```python
from build123d import *

# Parameters (mm, degrees)
BOSS_EXTRUDE1_DEPTH     = 10
BOSS_EXTRUDE2_DEPTH     = 30
BOSS_EXTRUDE3_REACH     = 323.598
CUT_EXTRUDE1_DEPTH      = 396.885084336
CUT_EXTRUDE1_DEPTH_BACK = 396.885084336
SKETCH5_W               = 30
SKETCH5_H               = 30


with BuildPart() as part:
    # Sketch1 → Boss-Extrude1 (new body)
    with BuildSketch(Plane(origin=(0, 0, 0), x_dir=(1, 0, 0), z_dir=(0, 1, 0))):
        with BuildLine():
            Line((-185, -65), (5, -65))
            ThreePointArc((5, -65), (60.514401442, -84.704810384), (91.182336182, -135))
            Line((91.182336182, -135), (185, -135))
            Line((185, -135), (185, 135))
            Line((185, 135), (-185, 135))
            Line((-185, 135), (-185, -65))
        make_face()
    extrude(amount=BOSS_EXTRUDE1_DEPTH)

    # Sketch2 → Boss-Extrude2 (add)
    with BuildSketch(Plane(origin=(0, 10, 0), x_dir=(1, 0, 0), z_dir=(0, 1, 0))):
        Polygon((-175, -35), (-175, 30), (-185, 30), (-185, -45), (-142.5, -45), (-142.5, -35), align=None)
        Polygon((-175, 125), (-142.5, 125), (-142.5, 135), (-185, 135), (-185, 60), (-175, 60), align=None)
        Polygon((-95, -35), (-95, 30), (-85, 30), (-85, -45), (-127.5, -45), (-127.5, -35), align=None)
        Polygon((-127.5, 135), (-127.5, 125), (-95, 125), (-95, 60), (-85, 60), (-85, 135), align=None)
    extrude(amount=BOSS_EXTRUDE2_DEPTH)

    # Boss-Extrude3: up to this face of the body (flat: up to its plane)
    boss_extrude3_end = Plane(part.part.faces().sort_by_distance((-158.75, 25, 35))[0])
    # Sketch3 → Boss-Extrude3 (add, up to the picked face)
    with BuildSketch(Plane.XY.offset(-125), mode=Mode.PRIVATE) as boss_extrude3_sk1:
        with BuildLine():
            ThreePointArc((-134.999999946, 10), (-159.999999978, 18.333333317), (-175, 40))
            Line((-175, 40), (-175, 10))
            Line((-175, 10), (-134.999999946, 10))
        make_face()
    boss_extrude3_tool1 = split(extrude(boss_extrude3_sk1.sketch, amount=BOSS_EXTRUDE3_REACH, mode=Mode.PRIVATE), bisect_by=boss_extrude3_end, keep=Keep.BOTH, mode=Mode.PRIVATE)
    # Sketch3 → Boss-Extrude3 (add, up to the picked face)
    with BuildSketch(Plane.XY.offset(-125), mode=Mode.PRIVATE) as boss_extrude3_sk2:
        with BuildLine():
            Line((-134.999999946, 10), (-95, 10))
            Line((-95, 10), (-95, 40))
            ThreePointArc((-95, 40), (-109.999999978, 18.33333335), (-134.999999946, 10))
        make_face()
    boss_extrude3_tool2 = split(extrude(boss_extrude3_sk2.sketch, amount=BOSS_EXTRUDE3_REACH, mode=Mode.PRIVATE), bisect_by=boss_extrude3_end, keep=Keep.BOTH, mode=Mode.PRIVATE)
    add(boss_extrude3_tool1.solids().sort_by(Axis((-165.840385, 17.926758, -125), (0, 0, 1)))[0])
    add(boss_extrude3_tool2.solids().sort_by(Axis((-104.159615, 17.926758, -125), (0, 0, 1)))[0])

    # Sketch5 → Cut-Extrude1 (cut, two sides: drawn at the far end of the back side and taken through both)
    with BuildSketch(Plane.ZY.offset(185).offset(-CUT_EXTRUDE1_DEPTH_BACK)):
        with Locations((-45, 25)):
            Rectangle(SKETCH5_W, SKETCH5_H)
    extrude(amount=CUT_EXTRUDE1_DEPTH + CUT_EXTRUDE1_DEPTH_BACK, mode=Mode.SUBTRACT)


solid = part.part
```
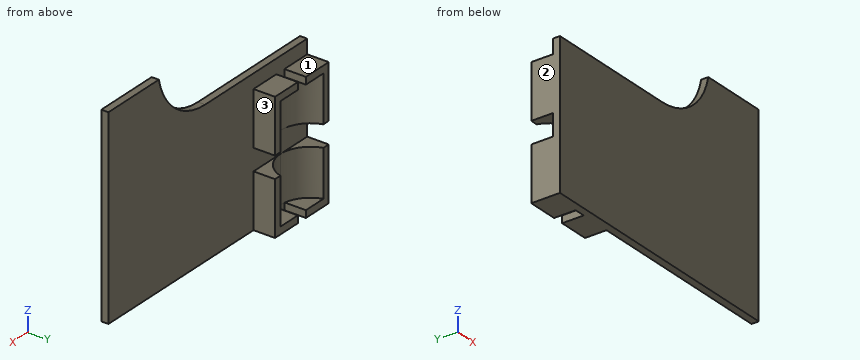
Geometry: final body of the model. Coordinates: model frame, mm. Face numbers are marked on the shaded views. A direction names the side the tool comes from. Coordinates: 2 decimals unless noted, no trailing zeros. Order: outer loops, then holes, each group sorted by start corner. A loop starts at its lowest first (then second) coordinate and runs counter-clockwise, first axis right, second up.
Item 1: Section query D-D (x = 79). Output: boundary loops of the cut face in (y, z), then the cut area to 3 significant figures.
Answer:
outline: (0, -135) - (10, -135) - (10, 105.33) - (0, 105.33) - close
area: 2,400 mm2
Item 2: Section query C-C (x = 118.5). Output: boundary loops of the cut face in (y, z).
Answer:
outline: (0, -135) - (10, -135) - (10, 135) - (0, 135) - close
Item 3: Access query for the marked faces 1, 2 and 3. Directions: +Z, -Z, +X, -X, +Y, -Y. A direction counts if a zero-diameter tool reaches every point of the face in a straight line with its end or side. Return the directions, or none.
Answer:
face 1: +Z, +X, -X, +Y
face 2: +Z, -Z, -X, +Y, -Y
face 3: +Z, -Z, +X, +Y
Item 4: Section query A-A (y = 26.5). Output: boundary loops of the cut face in (x, z), then the cut area to 3 significant figures.
Answer:
outline: (-185, -135) - (-142.5, -135) - (-142.5, -125) - (-168.21, -125) - (-168.21, -60) - (-185, -60) - close; (-185, -30) - (-168.21, -30) - (-168.21, 35) - (-142.5, 35) - (-142.5, 45) - (-185, 45) - close; (-127.5, -135) - (-85, -135) - (-85, -60) - (-101.79, -60) - (-101.79, -125) - (-127.5, -125) - close; (-127.5, 35) - (-101.79, 35) - (-101.79, -30) - (-85, -30) - (-85, 45) - (-127.5, 45) - close
area: 6,070 mm2
Item 5: Material intervals for line 1 along X through (y, z) = (17.5, 40.5); line 2 along Y through (x, z) = (162, 97.5); line 3 along Z through (x, y) = (-151, 3.5), sorted ascending.
Answer:
line 1: x = -185 to -142.5, -127.5 to -85
line 2: y = 0 to 10
line 3: z = -135 to 65
Item 6: Contact query for flat-ended pins moving along their axis: P1, Ø3, axis at x = -88.5, y = 6.5, coming from the +Z side; P2, Ø1, axis at x = -145.5, y = 34.5, coming from the +Z side; P3, Ø5, axis at y = 31.5, z = -129.5, coming from the +X side. Output: stop coordinate, or through.
Answer:
P1: stops at z = 65
P2: stops at z = 45
P3: stops at x = -85
Item 7: Section query B-B (z = -1). Output: boundary loops of the cut face in (x, y).
Answer:
outline: (-185, 0) - (185, 0) - (185, 10) - (-85, 10) - (-85, 40) - (-95, 40) arc R41.67 cw to (-175, 40) - (-185, 40) - close
